from build123d import *

# Parameters (mm, degrees)
F0_R     = 14.25
F1_DEPTH = 10
F2_R     = 16
F3_DEPTH = 2.5
F4_SIZE  = 1
F5_R     = 10.05
F6_DEPTH = 15


with BuildPart() as f1:
    # F0 (on Front) → F1 (new body)
    with BuildSketch(Plane.XZ):
        Circle(F0_R)
    extrude(amount=F1_DEPTH)

    # F2 (on Front) → F3 (join)
    with BuildSketch(Plane.XZ):
        Circle(F2_R)
    extrude(amount=-F3_DEPTH)

    # F4
    f4_edges = [f1.edges().sort_by_distance(p)[0] for p in [
        (-14.25, -10, 0),
    ]]
    chamfer(f4_edges, length=F4_SIZE)

    # F5 (on face) → F6 (cut)
    with BuildSketch(Plane.XZ.offset(10)):
        Circle(F5_R)
    extrude(amount=-F6_DEPTH, mode=Mode.SUBTRACT)


solid = f1.part
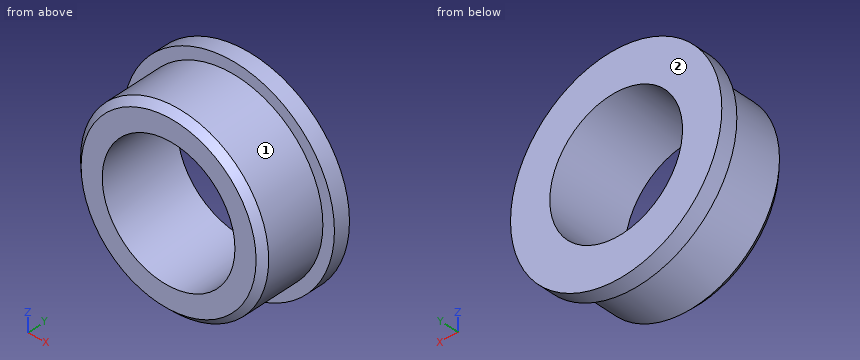
The listing builds one solid part. Answer for the finished solid, in the listing's coordinates (mm). Face numbers are marked on the shaded views. A direction names the side the tool comes from. Give positions to 0.01 mm unless a question says otherwise; leave off trailing zeros. Order: outer loops, then holes, each group sorted by start corner. A loop starts at its lowest first (then second) coordinate and runs counter-clockwise, first axis right, second up. Notation, with made-up numbers: (15.5, -10.5) - (70.5, -10.5) arc R16 cw to (70.5, 10.5) - close; hole circle Ø5 at (-30.5, -36). An arc over 180 degrees is marked (long way). Answer as CSV lines item,"result".
Q1. Each of these flat-tipped pins is pushed along its axis until it touches: pin 1 Ø4 at (x, y) = (-12.5, -5) entering from +Z; pin 2 Ø5 at (y, z) = (0.5, -11.5) entering from -X; pin 3 Ø3 at (y, z) = (-8.5, 4.5) entering from +X; pin 4 Ø9.5 at (x, z) = (1, -5) entering from -Y. Where does it stop, or does it pass through?
Answer key:
pin 1,"stops at z = 9.63"
pin 2,"stops at x = -13.23"
pin 3,"stops at x = 13.93"
pin 4,"passes through"
Q2. A cutting plane is placed at C-C, the plane y = -7. Determine the outline of the cut face in (x, z), and give its area (3 significant figures).
Answer key:
outline,"circle Ø28.5 at (0, 0); hole circle Ø20.1 at (0, 0)"
area,"321 mm^2"
Q3. A cutting plane is placed at B-B, the plane z = 0. Determine the outline of the cut face in (x, y), and give its area (3 significant figures).
Answer key:
outline,"(-16, 0) - (-14.25, 0) - (-14.25, -9) - (-13.25, -10) - (-10.05, -10) - (-10.05, 2.5) - (-16, 2.5) - close; (10.05, -10) - (13.25, -10) - (14.25, -9) - (14.25, 0) - (16, 0) - (16, 2.5) - (10.05, 2.5) - close"
area,"113 mm^2"
Q4. A cutting plane is placed at A-A, the plane x = 0. Determine the outline of the cut face in (y, z).
Answer key:
outline,"(-10, -13.25) - (-9, -14.25) - (0, -14.25) - (0, -16) - (2.5, -16) - (2.5, -10.05) - (-10, -10.05) - close; (-10, 10.05) - (2.5, 10.05) - (2.5, 16) - (0, 16) - (0, 14.25) - (-9, 14.25) - (-10, 13.25) - close"
Q5. Which of the six approach directions +Z, -Z, +X, -X, +Y, -Y give full straight-line access (tool end or side, diameter ignored) to the marked faces 1 and 2?
Answer key:
face 1,"-Y"
face 2,"+Z, -Z, +X, -X, +Y"
Q6. Straight lines are drawn through the part: L1, parallel to Z at x = 0, y = -5.5; L2, parallel to Z at x = 0, y = 2; L3, parallel to X at y = -3.75, z = 6. For each, find the intervals that lie inside material, in ascending order.
Answer key:
L1,"z = -14.25 to -10.05, 10.05 to 14.25"
L2,"z = -16 to -10.05, 10.05 to 16"
L3,"x = -12.93 to -8.06, 8.06 to 12.93"
